The model under review builds one solid part; all positions refer to its coordinate system, in mm. Give positions to 0.01 mm unless a question says otherwise; leave off trailing zeros. Loops run counter-clockwise (first coordinate to the right, second up) from the corner with the lowest first, then second, coordinate; pieces in that order, holes last. Notation, with made-up numbers: (18, 86.5) -> (50, 86.5) arc R9 cw to (50, 103.5) -> close; hole circle Ø4 at (19.25, 11.25). An arc over 180 degrees is marked (long way). Write each question's results on one line, items separated by ' | '. Start each with the question number.
Q1. We need section A-A (x = 0). Write out the cut boundary in (y, z), plus the area to 3 significant figures.
Q2. We need section D-D (z = -33). Write out the cut boundary in (x, y).
Q3. We need section C-C (z = 0). Write out the cut boundary in (x, y), plus the area to 3 significant figures.
Q4. Wall thickness on L1, parallel to X at y = 3.75, z = -3; L2, parallel to X at y = 3.5, z = -37; L3, parallel to X at y = 4, z = -67: over which ranges is each line inside the solid? List them lowest first. Write a range as [from, to].
Q5. Mouldability with a two-part tool opening along Z and no side actions: class faces 1 (the face through (0, -5, -47)), 2 (the face through (0.401, -4.84, 19.155)), 3 (the face through (-2.17, 0.06, -42.76)), 4 (the face through (-5.158, 0.056, -3.955)) as released by +Z, released by -Z, zero draft, split by the parting line, or undercut.
Q6. Insertion check: pin 1 Ø4 at (x, y) = (-6.5, 1) entering from -Z; pin 2 Ø5 at (y, z) = (-1, -76.5) entering from -X; pin 3 Ø2 at (x, z) = (4.5, -23) entering from -Y; pin 4 Ø8 at (x, z) = (0, 0) entering from -Y. Each pin has a flat end and moves straight along its axis. Give the tip position at first contact, or say it passes through.
Q7. We need section B-B (y = 2). Write out the cut boundary in (x, z), plus the area to 3 significant figures.
from build123d import *

# Parameters (mm, degrees)
F0_R     = 10
F0_R_2   = 6.5
F1_DEPTH = 5
F2_SIZE2 = 1
F2_SIZE  = 1
F3_SIZE2 = 1
F3_SIZE  = 1


with BuildPart() as f1:
    # F0 (on Front) → F1 (new body, symmetric)
    with BuildSketch(Plane.XZ):
        with BuildLine():
            Line((-19.942525, 1.515152), (-24.928157, -64.106061))
            ThreePointArc((-24.928157, -64.106061), (0, -91), (24.928157, -64.106061))
            Line((24.928157, -64.106061), (19.942525, 1.515152))
            ThreePointArc((19.942525, 1.515152), (0, 20), (-19.942525, 1.515152))
        make_face()
        with Locations((0, -33)):
            Circle(F0_R, mode=Mode.SUBTRACT)
        Circle(F0_R_2, mode=Mode.SUBTRACT)
    extrude(amount=F1_DEPTH, both=True)

    # F2
    f2_edges = [f1.edges().sort_by_distance(p)[0] for p in [
        (0, -5, 20),
        (-22.435341, -5, -31.295455),
        (0, -5, -91),
        (22.435341, -5, -31.295455),
        (-10, -5, -33),
        (-6.5, -5, 0),
    ]]
    chamfer(f2_edges, length=F2_SIZE, length2=F2_SIZE2)

    # F3
    f3_edges = [f1.edges().sort_by_distance(p)[0] for p in [
        (0, 5, 20),
        (-22.435341, 5, -31.295455),
        (0, 5, -91),
        (22.435341, 5, -31.295455),
        (-10, 5, -33),
        (-6.5, 5, 0),
    ]]
    chamfer(f3_edges, length=F3_SIZE, length2=F3_SIZE2)


solid = f1.part
Output:
1) outline: (-5, -90) -> (-4, -91) -> (4, -91) -> (5, -90) -> (5, -44) -> (4, -43) -> (-4, -43) -> (-5, -44) -> close; (-5, -22) -> (-4, -23) -> (4, -23) -> (5, -22) -> (5, -7.5) -> (4, -6.5) -> (-4, -6.5) -> (-5, -7.5) -> close; (-5, 7.5) -> (-4, 6.5) -> (4, 6.5) -> (5, 7.5) -> (5, 19) -> (4, 20) -> (-4, 20) -> (-5, 19) -> close | area: 774 mm2
2) outline: (-22.56, -4) -> (-21.56, -5) -> (-11, -5) -> (-10, -4) -> (-10, 4) -> (-11, 5) -> (-21.56, 5) -> (-22.56, 4) -> close; (10, -4) -> (11, -5) -> (21.56, -5) -> (22.56, -4) -> (22.56, 4) -> (21.56, 5) -> (11, 5) -> (10, 4) -> close
3) outline: (-20.06, -4) -> (-19.05, -5) -> (-7.5, -5) -> (-6.5, -4) -> (-6.5, 4) -> (-7.5, 5) -> (-19.05, 5) -> (-20.06, 4) -> close; (6.5, -4) -> (7.5, -5) -> (19.05, -5) -> (20.06, -4) -> (20.06, 4) -> (19.05, 5) -> (7.5, 5) -> (6.5, 4) -> close | area: 267 mm2
4) L1: [-20.29, -5.77], [5.77, 20.29] | L2: [-22.87, -9.17], [9.17, 22.87] | L3: [-24.98, 24.98]
5) face 1: zero draft | face 2: released by +Z | face 3: undercut | face 4: undercut
6) pin 1: z = -90.59 | pin 2: x = -23.69 | pin 3: y = -5 | pin 4: through
7) outline: (-24.93, -64.11) arc R25 ccw (long way) to (24.93, -64.11) -> (19.94, 1.52) arc R20 ccw to (-19.94, 1.52) -> close; hole circle Ø20 at (0, -33); hole circle Ø13 at (0, 0) | area: 4,140 mm2
